Answer from the drawing. Dimensions are ordinates in mm from the lowest x, y and z of the part. A direction names the side the tool comes from. Coordinates: 2 decimals unless noted, no trailing zeros. Write each loop counter-clockwise with the first axis right and the second up, starting at its lowest first coordinate (ties: lowest second). Pieces come first, ordered by that corner, then holes. Notation, with made-up numbers: (33, 56.25) - (39, 56.25) arc R4 cw to (39, 60.25) - close; hole circle Ø2 at (-16.75, 70.5). An arc over 180 degrees is marked (long way). Use CSV: the item, a comma, the result in double quotes. Start each with the question number.
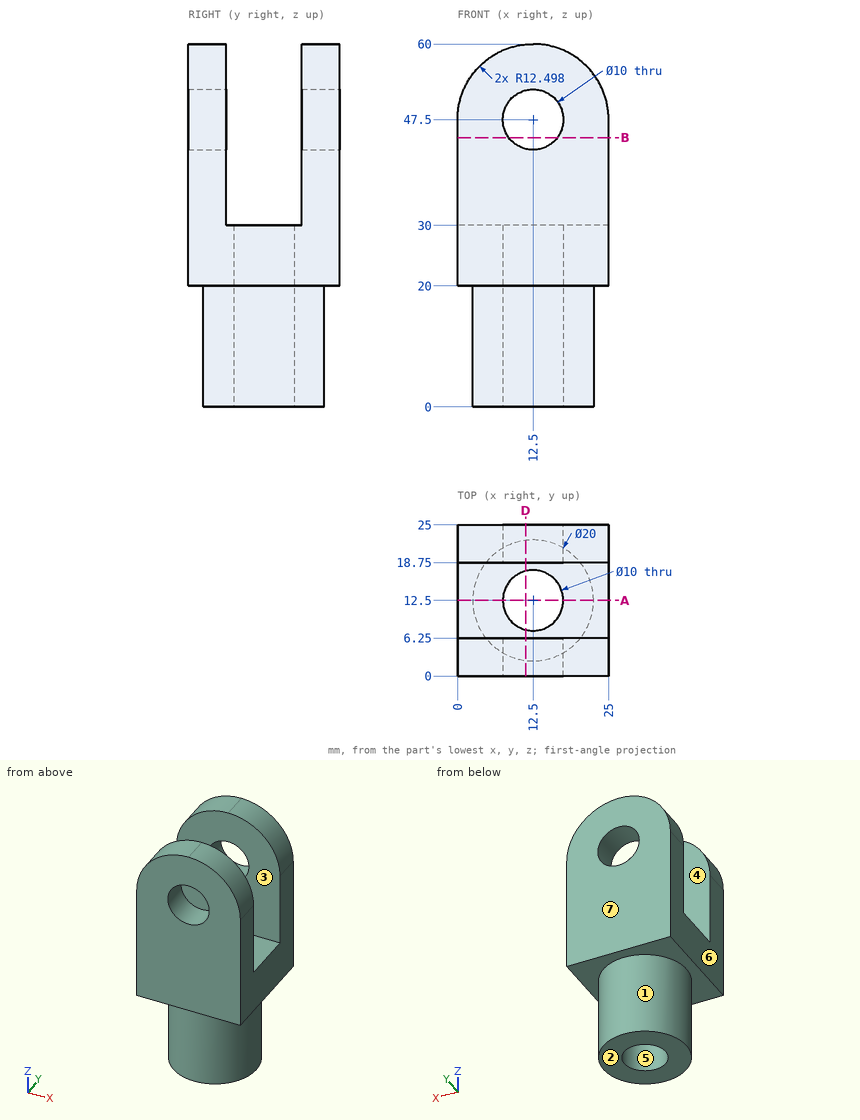
Item 1: Straight lines are drawn through the part: probe 1 along Y at (x, z) = (23, 47); probe 2 along Y at (x, z) = (12.5, 15); probe 3 along X at (y, z) = (12.25, 12). For each, find the intervals that lie inside material, in ascending order. Write a range as [from, to].
Item 2: Which of the six approach directions +Z, -Z, +X, -X, +Y, -Y give full straight-line access (tool end or side, diameter ignored) to the marked faces 1, 2 and 3?
Item 3: A cutting plane is placed at A-A (y = 12.5). Determine the outline of the cut face in (x, z).
Item 4: A cutting plane is placed at D-D (x = 11.25). Determine the outline of the cut face in (y, z).
Item 5: A cutting plane is placed at B-B (z = 44.5). Determine the outline of the cut face in (x, y).
Item 6: Each of these flat-tipped pins is pushed along its axis until it touches: pin 1 (12.5 mm diameter, centred on x = 8.5, z = 39.5, fed in from -Y); pin 2 (8 mm diameter, centred on x = 4, z = 8.5, fed in from -Y); pin 3 (6 mm diameter, centred on x = 8, y = 11, fed in from +Z); pin 4 (3 mm diameter, centred on x = 22, z = 7.5, fed in from -Y). Where does it stop, or does it pass through?
Item 7: Determine the mould class of the marked faces 4, 5, 6 and 7 for opening direction Y: +Y half, -Y half, draft (parallel to the pull), parting line (faces both ways), or undercut.
Calculated:
1,probe 1,"y = [0, 6.25], [18.75, 25]"
1,probe 2,"y = [2.5, 7.5], [17.5, 22.5]"
1,probe 3,"x = [2.5, 7.51], [17.49, 22.5]"
2,face 1,"-Z"
2,face 2,"-Z, +X, -X, +Y, -Y"
2,face 3,"+Z, +X, -X"
3,outline,"(0, 20) - (2.5, 20) - (2.5, 0) - (7.5, 0) - (7.5, 30) - (0, 30) - close; (17.5, 0) - (22.5, 0) - (22.5, 20) - (25, 20) - (25, 30) - (17.5, 30) - close"
4,outline,"(0, 20) - (2.58, 20) - (2.58, 0) - (7.66, 0) - (7.66, 30) - (6.25, 30) - (6.25, 42.66) - (0, 42.66) - close; (0, 52.34) - (6.25, 52.34) - (6.25, 59.94) - (0, 59.94) - close; (17.34, 0) - (22.42, 0) - (22.42, 20) - (25, 20) - (25, 42.66) - (18.75, 42.66) - (18.75, 30) - (17.34, 30) - close; (18.75, 52.34) - (25, 52.34) - (25, 59.94) - (18.75, 59.94) - close"
5,outline,"(0, 0) - (8.5, 0) - (8.5, 6.25) - (0, 6.25) - close; (0, 18.75) - (8.5, 18.75) - (8.5, 25) - (0, 25) - close; (16.5, 0) - (25, 0) - (25, 6.25) - (16.5, 6.25) - close; (16.5, 18.75) - (25, 18.75) - (25, 25) - (16.5, 25) - close"
6,pin 1,"stops at y = 0"
6,pin 2,"stops at y = 3.57"
6,pin 3,"stops at z = 30"
6,pin 4,"stops at y = 6.5"
7,face 4,"undercut"
7,face 5,"undercut"
7,face 6,"draft"
7,face 7,"+Y half"
